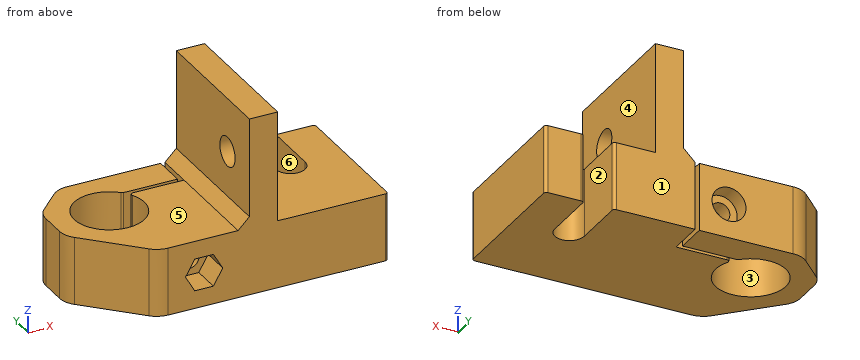
```python
from build123d import *

# Parameters (mm, degrees)
PAD_DEPTH       = 31.5
SKETCH001_W     = 20
SKETCH001_H     = 30
SKETCH001_W_2   = 27
POCKET_DEPTH    = 19.5
SKETCH002_R     = 2.6
POCKET001_DEPTH = 24.501
SKETCH003_R     = 1.7
POCKET002_DEPTH = 25.001
SKETCH004_R     = 3
POCKET003_DEPTH = 3
POCKET004_DEPTH = 5
CHAMFER_SIZE    = 2
FILLET_R        = 0.5


with BuildPart() as part:
    # Sketch → Pad (new body)
    with BuildSketch(Plane.XY):
        with BuildLine():
            ThreePointArc((-0.171573, -13.828427), (1.126121, -14.695518), (2.656854, -15))
            Line((41.00007, -14.999422), (2.656854, -15))
            ThreePointArc((41.00007, -14.999422), (41.353579, -14.85295), (41.5, -14.499421))
            Line((41.5, 9.5), (41.5, -14.499421))
            ThreePointArc((41.5, 9.5), (41.353578, 9.853528), (41.000071, 10))
            Line((34.6, 10), (41.000071, 10))
            Line((34.6, 10), (34.6, 0))
            ThreePointArc((29.4, 0), (32, -2.6), (34.6, 0))
            Line((29.4, 0), (29.4, 10))
            Line((15, 10), (29.4, 10))
            Line((15, 3.5), (15, 10))
            Line((5.990826, 3.5), (15, 3.5))
            ThreePointArc((5.990826, 3.5), (5.56542, 3.262735), (5.54375, 2.776119))
            ThreePointArc((4.372572, 4.395522), (-5.023841, -3.633322), (5.54375, 2.776119))
            ThreePointArc((4.372572, 4.395522), (4.534461, 4.28781), (4.725198, 4.25))
            Line((14.25, 4.25), (4.725198, 4.25))
            Line((14.25, 10), (14.25, 4.25))
            Line((-2.343146, 10), (14.25, 10))
            ThreePointArc((-2.343146, 10), (-3.873879, 9.695518), (-5.171573, 8.828427))
            Line((-5.171573, 8.828427), (-8.828427, 5.171573))
            ThreePointArc((-8.828427, 5.171573), (-9.695518, 3.873879), (-10, 2.343146))
            Line((-10, -2.343146), (-10, 2.343146))
            ThreePointArc((-10, -2.343146), (-9.695518, -3.873879), (-8.828427, -5.171573))
            Line((-8.828427, -5.171573), (-0.171573, -13.828427))
        make_face()
    extrude(amount=PAD_DEPTH)

    # Sketch001 (on Face26 of Pad) → Pocket (cut)
    with BuildSketch(Plane.XY.offset(31.5)):
        with Locations((32, 0)):
            Rectangle(SKETCH001_W, SKETCH001_H)
        with Locations((3.5, 0)):
            Rectangle(SKETCH001_W_2, SKETCH001_H)
    extrude(amount=-POCKET_DEPTH, mode=Mode.SUBTRACT)

    # Sketch002 (on Face29 of Pocket) → Pocket001 (cut, through all)
    with BuildSketch(Plane(origin=(17, 0, 0), x_dir=(0, -1, 0), z_dir=(-1, 0, 0))):
        with Locations((7.5, 22)):
            Circle(SKETCH002_R)
    extrude(amount=-POCKET001_DEPTH, mode=Mode.SUBTRACT)

    # Sketch003 (on Face13 of Pocket001) → Pocket002 (cut, through all)
    with BuildSketch(Plane(origin=(0, 10, 0), x_dir=(-1, 0, 0), z_dir=(0, 1, 0))):
        with Locations((-9, 6)):
            Circle(SKETCH003_R)
    extrude(amount=-POCKET002_DEPTH, mode=Mode.SUBTRACT)

    # Sketch004 (on Face13 of Pocket002) → Pocket003 (cut)
    with BuildSketch(Plane(origin=(0, 10, 0), x_dir=(-1, 0, 0), z_dir=(0, 1, 0))):
        with Locations((-9, 6)):
            Circle(SKETCH004_R)
    extrude(amount=-POCKET003_DEPTH, mode=Mode.SUBTRACT)

    # Sketch005 (on Face21 of Pocket003) → Pocket004 (cut)
    with BuildSketch(Plane(origin=(0.000226, -15.00004, 0), x_dir=(1, 1.5e-05, 0), z_dir=(1.5e-05, -1, 0))):
        Polygon((10.645448, 3.15), (12.290897, 6), (10.645448, 8.85), (7.354552, 8.85), (5.709103, 6), (7.354552, 3.15), align=None)
    extrude(amount=-POCKET004_DEPTH, mode=Mode.SUBTRACT)

    # Chamfer
    chamfer_edges = [part.edges().sort_by_distance(p)[0] for p in [
        (17, -2.499892, 12),
    ]]
    chamfer(chamfer_edges, length=CHAMFER_SIZE)

    # Fillet
    fillet_edges = [part.edges().sort_by_distance(p)[0] for p in [
        (34.6, 10, 6),
        (29.4, 10, 6),
    ]]
    fillet(fillet_edges, radius=FILLET_R)


solid = part.part
```
The listing builds one solid part. Answer for the finished solid, in the listing's coordinates (mm). Face numbers are marked on the shaded views. A direction names the side the tool comes from. Round coordinates to 2 decimals unless told otherwise and drop trailing zeros. Loops run counter-clockwise (first coordinate to the right, second up) from the corner with the lowest first, then second, coordinate; pieces in that order, holes last.
1) A cutting plane is placed at C-C on z = 26.5. Determine the outline of the cut face in (x, y).
Outcome:
outline: (17, -15) - (22, -15) - (22, 10) - (17, 10) - close
2) A cutting plane is placed at D-D on x = 30. Determine the outline of the cut face in (y, z).
Outcome:
outline: (-15, 0) - (-1.66, 0) - (-1.66, 12) - (-15, 12) - close
3) For a pull along Y with two mould halves and no side action, classify the marked faces 1, 2 and 3 as released by +Y, released by -Y, zero draft, split by the parting line, or undercut.
Outcome:
face 1: released by +Y
face 2: zero draft
face 3: undercut
4) For the marked faces 4, 5 and 6, determine the directions among +Z, -Z, +X, -X, +Y, -Y from which every point of the face is accessible in a straight line to the end or side of a thin tool.
Outcome:
face 4: +Z, +X, +Y, -Y
face 5: +Z, -X, +Y, -Y
face 6: +Z, -Z, +Y
5) Given P1, Ø6, axis at x = 27, y = -4.5, coming from the +Z side; P2, Ø3, axis at y = -12, z = 28, coming from the +X side; P3, Ø1.5, axis at x = -3.5, z = 9.5, coming from the +Y side; P4, Ø7.5, axis at x = 0, y = 0, coming from the +Z side, each flat-ended and moving along its own axis, determine where each tip first touches the part or whether it passes through.
Outcome:
P1: stops at z = 12
P2: stops at x = 22
P3: stops at y = 9.98
P4: passes through
6) Consider line 1 (X direction, y = 0, z = 8.5); line 2 (Z direction, x = 9, y = 5.4); line 3 (Y direction, x = 10, z = 1). Determine where each line is inside the solid, lowest interval first.
Outcome:
line 1: x = -10 to -6.2, 6.2 to 29.4, 34.6 to 41.5
line 2: z = 0 to 4.3, 7.7 to 12
line 3: y = -15 to 3.5, 4.25 to 10
7) A cutting plane is placed at A-A on z = 23. Determine the outline of the cut face in (x, y).
Outcome:
outline: (17, -15) - (22, -15) - (22, -9.9) - (17, -9.9) - close; (17, -5.1) - (22, -5.1) - (22, 10) - (17, 10) - close
8) A cutting plane is placed at B-B on x = 9. Determine the outline of the cut face in (y, z), plus the area to 3 significant figures.
Outcome:
outline: (-15, 0) - (3.5, 0) - (3.5, 4.3) - (-10, 4.3) - (-10, 3.15) - (-15, 3.15) - close; (-15, 8.85) - (-10, 8.85) - (-10, 7.7) - (3.5, 7.7) - (3.5, 12) - (-15, 12) - close; (4.25, 0) - (10, 0) - (10, 3) - (7, 3) - (7, 4.3) - (4.25, 4.3) - close; (4.25, 7.7) - (7, 7.7) - (7, 9) - (10, 9) - (10, 12) - (4.25, 12) - close
area: 189 mm2
